```python
from build123d import *

# Parameters (mm, degrees)
F1_DEPTH = 24
F3_DEPTH = 20


with BuildPart() as f1:
    # F0 (on Top) → F1 (new body)
    with BuildSketch(Plane.XY):
        with BuildLine():
            Line((-1.58542, 17.428036), (-14, 40))
            Line((-14, 40), (-50, 40))
            Line((-50, 40), (-50, -40))
            Line((-50, -40), (30, -40))
            Line((30, -40), (13.869489, -10.671798))
            ThreePointArc((13.869489, -10.671798), (-15.333778, -8.433578), (-1.58542, 17.428036))
        make_face()
        with BuildLine():
            Line((50, -40), (50, 40))
            Line((50, 40), (-14, 40))
            Line((-14, 40), (-1.58542, 17.428036))
            ThreePointArc((-1.58542, 17.428036), (11.800533, 12.922748), (17.5, 0))
            ThreePointArc((17.5, 0), (16.567529, -5.63622), (13.869489, -10.671798))
            Line((13.869489, -10.671798), (30, -40))
            Line((30, -40), (50, -40))
        make_face()
    extrude(amount=F1_DEPTH)

    # F2 (on face) → F3 (join)
    with BuildSketch(Plane.XY.offset(24)):
        with BuildLine():
            Line((50, 40), (-30, 40))
            Line((-30, 40), (-13.869489, 10.671798))
            ThreePointArc((-13.869489, 10.671798), (5.63622, 16.567529), (17.5, 0))
            ThreePointArc((17.5, 0), (12.922748, -11.800533), (1.58542, -17.428036))
            Line((1.58542, -17.428036), (14, -40))
            Line((14, -40), (50, -40))
            Line((50, -40), (50, 40))
        make_face()
    extrude(amount=F3_DEPTH)


solid = f1.part
```
Geometry: final body of the model. Coordinates: model frame, mm. A direction names the side the tool comes from. Coordinates: 2 decimals unless noted, no trailing zeros. Loops run counter-clockwise (first coordinate to the right, second up) from the corner with the lowest first, then second, coordinate; pieces in that order, holes last. Notation, with made-up numbers: M 22.25,19.5 L 26.25,19.5 A13 ccw 26.25,39.5 Z; hole C 45,-32 d6. An arc over 180 degrees is marked long. Put each result on its own line as item: value.
(1) Cut plane A-A on x = 0. Return the cut outline in (y, z), then the cut area to 3 significant figures.
Answer sheet:
outline: M -40,0 L -17.5,0 L -17.5,24 L -40,24 Z; M 17.5,0 L 40,0 L 40,44 L 17.5,44 Z
area: 1,530 mm^2
(2) Cut plane B-B on z = 11. Return the cut outline in (x, y).
Answer sheet:
outline: M -50,-40 L 50,-40 L 50,40 L -50,40 Z; hole M 13.87,-10.67 A17.5 ccw 17.5,0 A17.5 ccw long Z
(3) Material intervals for probe 1 along X at (y, z) = (0, 7.75); probe 2 along Y at (x, z) = (0, 18.5); probe 3 along Z at (x, y) = (-45, -5.5), sorted ascending.
Answer sheet:
probe 1: x = -50 to -17.5, 17.5 to 50
probe 2: y = -40 to -17.5, 17.5 to 40
probe 3: z = 0 to 24
(4) First-contact query: pin 1 (1 mm diameter, centred on y = 29.5, z = 38, fed in from -X). Flat tip, straight axial feed; report the tip coordinate or a pass-through.
Answer sheet:
pin 1: stops at x = -24.5
(5) Cut plane C-C on y = 12.5. Return the cut outline in (x, z) (3 decimals).
Answer sheet:
outline: M -50,0 L -12.247,0 L -12.247,44 L -14.875,44 L -14.875,24 L -50,24 Z; M 12.247,0 L 50,0 L 50,44 L 12.247,44 Z
(6) Access query for faces 1 (the face through (-22.048, 25.541, 33.86)), 2 (the face through (1, 40, 22)). Directions: +Z, -Z, +X, -X, +Y, -Y. A direction counts if a zero-diameter tool reaches every point of the face in a straight line with its end or side. Return the directions, or none.
Answer sheet:
face 1: +Z, -X, -Y
face 2: +Z, -Z, +X, -X, +Y
(7) Cut plane D-D on y = 32. Return the cut outline in (x, z), then the cut area to 3 significant figures.
Answer sheet:
outline: M -50,0 L 50,0 L 50,44 L -25.6,44 L -25.6,24 L -50,24 Z
area: 3,910 mm^2
